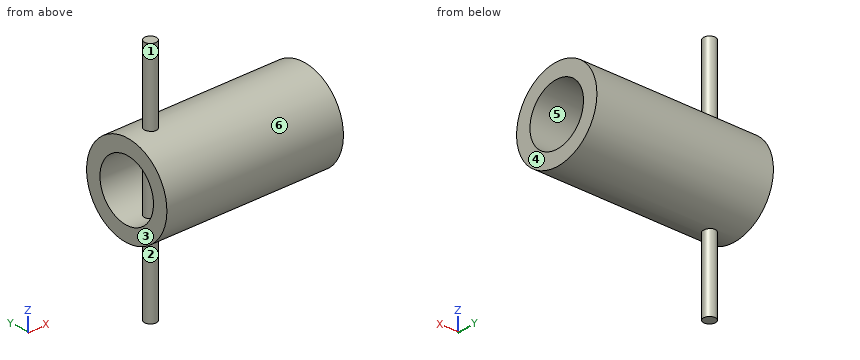
```python
from build123d import *

# Parameters (mm, degrees)
SKETCH1_R           = 37.5
SKETCH1_R_2         = 25
BOSS_EXTRUDE1_DEPTH = 75
SKETCH2_R           = 5
BOSS_EXTRUDE2_DEPTH = 100


with BuildPart() as part:
    # Sketch1 → Boss-Extrude1 (new body, symmetric)
    with BuildSketch(Plane(origin=(0, 0, 0), x_dir=(0, 0, -1), z_dir=(1, 0, 0))):
        Circle(SKETCH1_R)
        Circle(SKETCH1_R_2, mode=Mode.SUBTRACT)
    extrude(amount=BOSS_EXTRUDE1_DEPTH, both=True)

    # Sketch2 → Boss-Extrude2 (add, symmetric)
    with BuildSketch(Plane.XY):
        with Locations((-54.825376389, 0)):
            Circle(SKETCH2_R)
    extrude(amount=BOSS_EXTRUDE2_DEPTH, both=True)


solid = part.part
```
Design review of the part built by this model. Coordinates are the model's own, in mm. Face numbers are marked on the shaded views. A direction names the side the tool comes from. Coordinates: 2 decimals unless noted, no trailing zeros. Order: outer loops, then holes, each group sorted by start corner. A loop starts at its lowest first (then second) coordinate and runs counter-clockwise, first axis right, second up. Notation, with made-up numbers: (7.5, -36.5) - (12.5, -36.5) arc R27 ccw to (12.5, -8.5) - close; hole circle Ø7 at (88, 72). An arc over 180 degrees is marked (long way). One line per question, with ' | ' between items.
Q1. To check wall thickness, follow line 1 along Z through (x, y) = (-21.5, 0); line 2 along Z through (x, y) = (-33, -21). State the ranges of each line that lie inside material, in increasing order.
Answer key:
line 1: z = -37.5 to -25, 25 to 37.5 | line 2: z = -31.07 to -13.56, 13.56 to 31.07
Q2. For the marked faces 1, 2 and 3, list the 3-axis set-ups (+Z, -Z, +X, -X, +Y, -Y) from which the entire face can be reached by the end or side of a thin tool; tool diameter is ignored.
Answer key:
face 1: +Z | face 2: -Z | face 3: +Z, -Z, -X, +Y, -Y
Q3. Clearance check with flat-ended pins moving along their axes: pin 1 Ø1 at (x, z) = (-50, 43) entering from +Y; pin 2 Ø10 at (x, z) = (-22.5, 6.5) entering from -Y; pin 3 Ø8 at (x, y) = (45, -14) entering from +Z. State where each tip first meets the part, or that it passes through.
Answer key:
pin 1: stops at y = 2.51 | pin 2: stops at y = -37.47 | pin 3: stops at z = 36.14
Q4. The part is to be moulded in two halves that separate along Z. For the marked faces 4, 5 and 6, say which applies: +Z half, -Z half, draft (parallel to the pull), parting line (faces both ways), or undercut.
Answer key:
face 4: draft | face 5: undercut | face 6: parting line
Q5. Consider section A-A, the plane z = 0. Give the boundary of the cut face in (x, y), then the cut area to 3 significant figures.
Answer key:
outline: (-75, -37.5) - (75, -37.5) - (75, -25) - (-75, -25) - close; (-75, 25) - (75, 25) - (75, 37.5) - (-75, 37.5) - close; circle Ø10 at (-54.83, 0) | area: 3,830 mm2
Q6. Consider section C-C, the plane x = 21.5. Give the boundary of the cut face in (y, z).
Answer key:
outline: circle Ø75 at (0, 0); hole circle Ø50 at (0, 0)
Q7. Consider section D-D, the plane y = 0. Give the boundary of the cut face in (x, z), then the cut area to 3 significant figures.
Answer key:
outline: (-75, -37.5) - (-59.83, -37.5) - (-59.83, -100) - (-49.83, -100) - (-49.83, -37.5) - (75, -37.5) - (75, -25) - (-49.83, -25) - (-49.83, 25) - (75, 25) - (75, 37.5) - (-49.83, 37.5) - (-49.83, 100) - (-59.83, 100) - (-59.83, 37.5) - (-75, 37.5) - (-75, 25) - (-59.83, 25) - (-59.83, -25) - (-75, -25) - close | area: 5,500 mm2
Q8. Consider section B-B, the plane y = 18.5. Give the boundary of the cut face in (x, z), then the cut area to 3 significant figures.
Answer key:
outline: (-75, -32.62) - (75, -32.62) - (75, -16.82) - (-75, -16.82) - close; (-75, 16.82) - (75, 16.82) - (75, 32.62) - (-75, 32.62) - close | area: 4,740 mm2
